For this review, take the finished solid that the model builds, in its own axes (mm). Coordinates: 2 decimals unless noted, no trailing zeros. Write each loop counter-clockwise with the first axis right and the second up, starting at its lowest first coordinate (ties: lowest second). Pieces come first, ordered by that corner, then holes.
```python
from build123d import *

# Parameters (mm, degrees)
F0_W     = 32.004
F0_H     = 83.82
F1_DEPTH = 6.35
F3_D     = 30.48


with BuildPart() as f1:
    # F0 (on Top) → F1 (new body)
    with BuildSketch(Plane.XY):
        Polygon((-44.196, -76.2), (44.196, -76.2), (44.196, 7.62), (76.2, 7.62), (76.2, 76.2), (-76.2, 76.2), (-76.2, 7.62), (-44.196, 7.62), align=None)
        with Locations((-60.198, -34.29)):
            Rectangle(F0_W, F0_H)
        with Locations((60.198, -34.29)):
            Rectangle(F0_W, F0_H)
    extrude(amount=F1_DEPTH)

    # F3 (through all)
    with Locations(Plane.XY.offset(6.35)):
        with Locations((-44.196, 7.62), (44.196, 7.62)):
            Hole(F3_D / 2)


solid = f1.part
```
Q1. Add section C-C (y = 7.62). State the section outline as (x, z) points, then the cut area to 3 significant figures.
Ans:
outline: (-76.2, 0) - (-59.44, 0) - (-59.44, 6.35) - (-76.2, 6.35) - close; (-28.96, 0) - (28.96, 0) - (28.96, 6.35) - (-28.96, 6.35) - close; (59.44, 0) - (76.2, 0) - (76.2, 6.35) - (59.44, 6.35) - close
area: 581 mm2
Q2. Draft analysis for pull direction X (two halves, no side actions). For faces 1 (the cylindrical face through (-32.1, -1.65, 3.13)), 2 (the flat face through (76.2, -1, 3)), 3 (the flat face through (-1, 1, 6.35)), state which applies: +X half, -X half, draft (parallel to the pull), parting line (faces both ways), or undercut.
Ans:
face 1: undercut
face 2: +X half
face 3: draft
Q3. Clearance check with a flat-ended pin moving along its axis: pin 1 Ø18.5 at (x, y) = (44.196, 7.62) entering from +Z. State where the tip first meets the part, or that it passes through.
Ans:
pin 1: passes through
Q4. For probe 1 along X at (y, z) = (7.5, 5); probe 2 along X at (y, z) = (19.5, 5.25); probe 3 along Y at (x, z) = (-48, 4), list the stretches that pass through material, from the lowest coordinate up.
Ans:
probe 1: x = -76.2 to -59.44, -28.96 to 28.96, 59.44 to 76.2
probe 2: x = -76.2 to -53.74, -34.65 to 34.65, 53.74 to 76.2
probe 3: y = -76.2 to -7.14, 22.38 to 76.2
Q5. Add section B-B (x = 50.5). State the section outline as (y, z) points, then the cut area to 3 significant figures.
Ans:
outline: (-76.2, 0) - (-6.26, 0) - (-6.26, 6.35) - (-76.2, 6.35) - close; (21.5, 0) - (76.2, 0) - (76.2, 6.35) - (21.5, 6.35) - close
area: 792 mm2
Q6. Add section A-A (z = 3.5). State the section outline as (x, y) points.
Ans:
outline: (-76.2, -76.2) - (76.2, -76.2) - (76.2, 76.2) - (-76.2, 76.2) - close; hole circle Ø30.48 at (-44.2, 7.62); hole circle Ø30.48 at (44.2, 7.62)
